Design review of the part shown in the three views and the two pictorial views. Dimensions are in mm from the part's minimum x, y and z. Coordinates: 2 decimals unless noted, no trailing zeros. Write each loop counter-clockwise with the first axis right and the second up, starting at its lowest first coordinate (ties: lowest second). Pieces come first, ordered by that corner, then holes. Notation, with made-up numbers: (26.5, 44) - (59.5, 44) arc R15 ccw to (59.5, 64) - close; hole circle Ø7 at (-13, 88.5). An arc over 180 degrees is marked (long way). Return JSON: item names as keys, results as strings. Group by question number.
(1) To check wall thickness, follow L1, parallel to Y at x = 7, z = 20; L2, parallel to Z at x = 2.75, y = 43; L3, parallel to Y at x = 6.75, z = 17. State the ranges of each line that lie inside material, in increasing order. Write a range as from..to.
(2) We need section A-A on y = 30. State the section outline as (x, z) points.
(3) For pin 1 Ø2 at (y, z) = (43, 6.5) entering from -X; pin 2 Ø3 at (y, z) = (15.86, 34.14) entering from +X, all flat-tipped, find the tip position at first contact; note any pin that passes through.
(4) Draft analysis for pull direction Y (two halves, no side actions). For the marked faces 1, 2 and 3, state which applies: released by +Y, released by -Y, zero draft, split by the parting line, or undercut.
(5) We need section D-D on y = 41.5. State the section outline as (x, z) points, then the cut area to 3 significant figures.
(6) We need section B-B on z = 20. State the section outline as (x, y) points, then the cut area to 3 significant figures.
(7) We need section C-C on x = 3.5. State the section outline as (y, z) points.
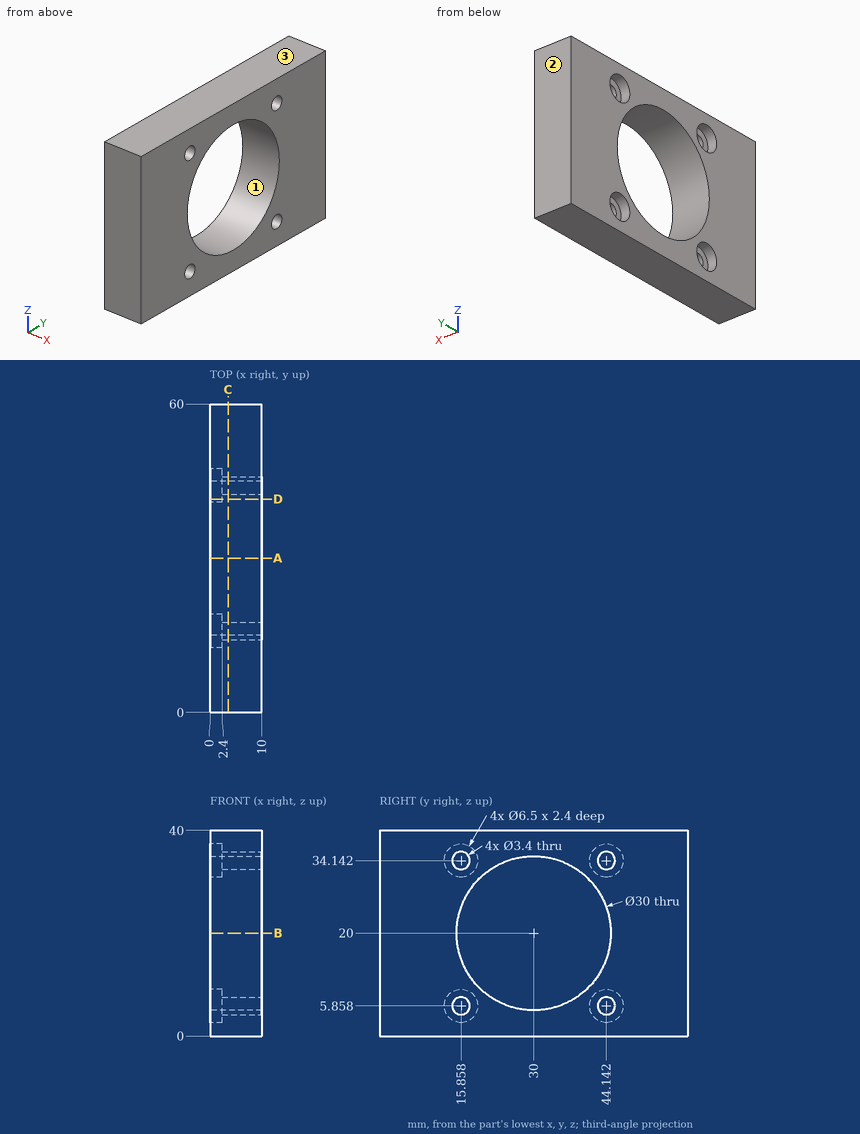
Ans:
{
 "1": {"L1": "0..15, 45..60", "L2": "0..4.6, 7.12..12.52, 27.48..32.88, 35.4..40", "L3": "0..15.3, 44.7..60"},
 "2": {"outline": "(0, 0) - (10, 0) - (10, 5) - (0, 5) - close; (0, 35) - (10, 35) - (10, 40) - (0, 40) - close"},
 "3": {"pin 1": "x = 2.4", "pin 2": "through"},
 "4": {"face 1": "undercut", "face 2": "released by +Y", "face 3": "zero draft"},
 "5": {"outline": "(0, 0) - (10, 0) - (10, 10.37) - (0, 10.37) - (0, 7.75) - (2.4, 7.75) - (2.4, 3.97) - (0, 3.97) - close; (0, 29.63) - (10, 29.63) - (10, 40) - (0, 40) - (0, 36.03) - (2.4, 36.03) - (2.4, 32.25) - (0, 32.25) - close", "area": "189 mm²"},
 "6": {"outline": "(0, 0) - (10, 0) - (10, 15) - (0, 15) - close; (0, 45) - (10, 45) - (10, 60) - (0, 60) - close", "area": "300 mm²"},
 "7": {"outline": "(0, 0) - (60, 0) - (60, 40) - (0, 40) - close; hole circle Ø3.4 at (15.86, 5.86); hole circle Ø3.4 at (15.86, 34.14); hole circle Ø30 at (30, 20); hole circle Ø3.4 at (44.14, 5.86); hole circle Ø3.4 at (44.14, 34.14)"}
}
